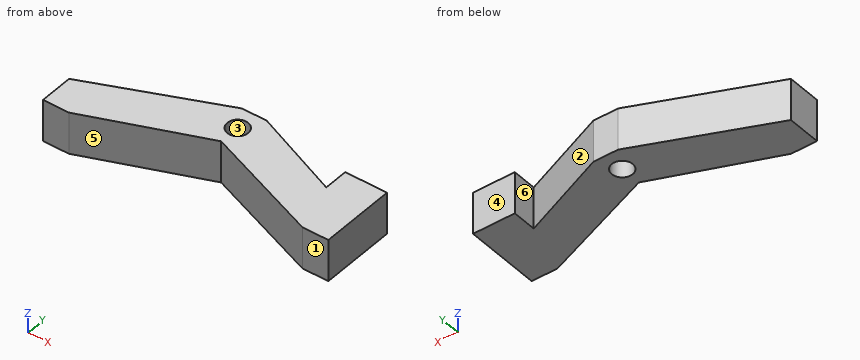
```python
from build123d import *

# Parameters (mm, degrees)
SKETCH1_R           = 2.5
BOSS_EXTRUDE1_DEPTH = 5
BOSS_EXTRUDE2_DEPTH = 10


with BuildPart() as part:
    # Sketch1 → Boss-Extrude1 (new, symmetric)
    with BuildSketch(Plane.XY):
        Polygon((0, 0), (27.955990735, -10.884051729), (34.143878012, -10.884051729), (34.143878012, -2.884051729), (2.966226636, 10.176810065), (-2.966226636, 10.176810065), (-34.143878012, -2.884051729), (-34.143878012, -10.884051729), (-27.955990735, -10.884051729), align=None)
        with Locations((0, 5.088405032)):
            Circle(SKETCH1_R, mode=Mode.SUBTRACT)
    extrude(amount=BOSS_EXTRUDE1_DEPTH, both=True)

    # Sketch3 → Boss-Extrude2 (add)
    with BuildSketch(Plane.XY.offset(5)):
        Polygon((34.143878012, -2.884051729), (24.143878012, 1.305122637), (24.143878012, 7.115948271), (34.143878012, 7.115948271), align=None)
    extrude(amount=-BOSS_EXTRUDE2_DEPTH)


solid = part.part
```
Here's how the part is built. I have some questions about the finished solid (model axes, mm). Face numbers are marked on the shaded views. A direction names the side the tool comes from. Give positions to 0.01 mm unless a question says otherwise; leave off trailing zeros. Loops run counter-clockwise (first coordinate to the right, second up) from the corner with the lowest first, then second, coordinate; pieces in that order, holes last. Notation, with made-up numbers: (12, -30) -> (42, -30) arc R28 ccw to (42, 3) -> close; hole circle Ø3 at (20.5, 58.5). An arc over 180 degrees is marked (long way). Use one line per item in the form item = value. Start each with the question number.
1) Thinking about a two-plate mould opening in Y: for the marked faces 1, 2 and 3, which applies, +Y half, -Y half, draft (parallel to the pull), parting line (faces both ways), or undercut?
2) Imagine slicing it at A-A (z = -2.5). Please give me the cut outline in (x, y).
3) Imagine slicing it at C-C (y = 4.5). Please give me the cut outline in (x, z).
4) For P1, Ø6.5, axis at x = 0, y = 5.09, coming from the -Z side; P2, Ø5, axis at y = 5, z = -2.5, coming from the -X side; P3, Ø1, axis at x = 10, z = 2, coming from the +Y side; P4, Ø1.7, axis at y = 5.5, z = 1.5, coming from the -X side, each with a flat end and sliding along its axis, tell me the tip position at first contact or that it passes through.
5) Imagine slicing it at D-D (x = -11). Please give me the cut outline in (y, z), then the cut area to 3 significant figures.
6) Please list where these lines run through material, in increasing order: line 1 along Y through (x, z) = (0, -0.5); line 2 along X through (y, z) = (6.5, -0.25); line 3 along X through (y, z) = (6.75, -4.5).
7) Which directions (+Z, -Z, +X, -X, +Y, -Y) give clear straight access to the entire face, cutting with the end or side of a thin tool? Please do the marked faces 4, 5 and 6.
8) Imagine slicing it at B-B (y = -8). Please give me the cut outline in (x, z).
Check values:
q1.face_1 = -Y half
q1.face_2 = +Y half
q1.face_3 = undercut
q2.outline = (-34.14, -10.88) -> (-27.96, -10.88) -> (0, 0) -> (27.96, -10.88) -> (34.14, -10.88) -> (34.14, 7.12) -> (24.14, 7.12) -> (24.14, 1.31) -> (2.97, 10.18) -> (-2.97, 10.18) -> (-34.14, -2.88) -> close; hole circle Ø5 at (0, 5.09)
q3.outline = (-16.52, -5) -> (-2.43, -5) -> (-2.43, 5) -> (-16.52, 5) -> close; (2.43, -5) -> (16.52, -5) -> (16.52, 5) -> (2.43, 5) -> close; (24.14, -5) -> (34.14, -5) -> (34.14, 5) -> (24.14, 5) -> close
q4.P1 = -5
q4.P2 = -21.29
q4.P3 = 7.44
q4.P4 = -16.16
q5.outline = (-4.28, -5) -> (6.81, -5) -> (6.81, 5) -> (-4.28, 5) -> close
q5.area = 111 mm^2
q6.line_1 = 0 to 2.59, 7.59 to 10.18
q6.line_2 = -11.74 to -2.06, 2.06 to 11.74, 24.14 to 34.14
q6.line_3 = -11.15 to -1.87, 1.87 to 11.15, 24.14 to 34.14
q7.face_4 = +Z, -Z, +X, +Y
q7.face_5 = +Z, -Z, -Y
q7.face_6 = +Z, -Z, +Y
q8.outline = (-34.14, -5) -> (-20.55, -5) -> (-20.55, 5) -> (-34.14, 5) -> close; (20.55, -5) -> (34.14, -5) -> (34.14, 5) -> (20.55, 5) -> close
